Geometry check sheet. Reference: the model listing, model coordinates, mm. Face numbers are marked on the shaded views. A direction names the side the tool comes from. Round coordinates to 2 decimals unless told otherwise and drop trailing zeros. Loops run counter-clockwise (first coordinate to the right, second up) from the corner with the lowest first, then second, coordinate; pieces in that order, holes last. Notation, with made-up numbers: (-13.75, 58.25) - (31.25, 58.25) arc R18 cw to (31.25, 75.25) - close; hole circle Ø11 at (-9, -4.75). An arc over 180 degrees is marked (long way). Answer in a Markdown table with one row per item. Add a question column.
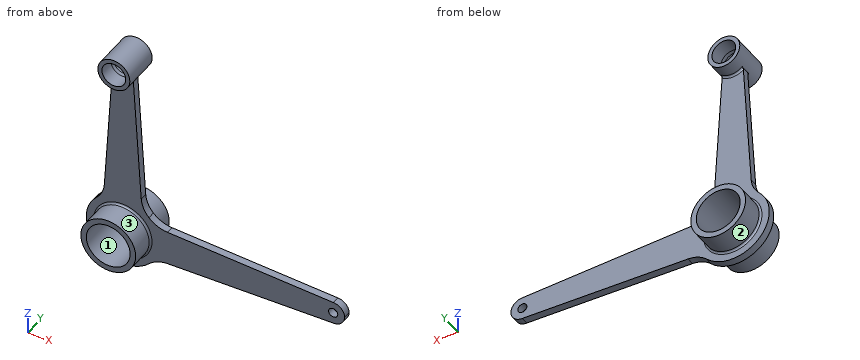
```python
from build123d import *

# Parameters (mm, degrees)
F0_R          = 30
F0_R_2        = 5
F0_R_3        = 13
F1_DEPTH      = 4
F2_R          = 30
F3_T1_DEPTH   = 8
F4_R          = 30
F5_R          = 30
F7_DEPTH      = 20
F6_R          = 30
F6_R_2        = 24
F8_DEPTH      = 30
F9_R          = 2
F10_T4_ANGLE  = 114.9160729666
F10_T10_ANGLE = 114.9160729666


# Not quite as in the source:
# - a fillet or chamfer that OpenCascade refuses, or shapes differently, is made with other operations: its cross-section is extruded or revolved along the edge and cut away or added


with BuildPart() as f1:
    # F0 (on Front) → F1 (new body, symmetric)
    with BuildSketch(Plane.XZ):
        with BuildLine():
            ThreePointArc((34.9249194702, -19.5), (38.7104428986, -10.074800772), (40, 0))
            ThreePointArc((40, 0), (38.7104428986, 10.074800772), (34.9249194702, 19.5))
            ThreePointArc((34.9249194702, 19.5), (28.892590505, 27.6625778609), (21, 34.0440890611))
            ThreePointArc((21, 34.0440890611), (0, 40), (-21, 34.0440890611))
            ThreePointArc((-21, 34.0440890611), (-27.6625778609, -28.892590505), (34.9249194702, -19.5))
        make_face()
        Circle(F0_R, mode=Mode.SUBTRACT)
        with BuildLine():
            ThreePointArc((34.9249194702, 19.5), (38.7104428986, 10.074800772), (40, 0))
            ThreePointArc((40, 0), (38.7104428986, -10.074800772), (34.9249194702, -19.5))
            Line((34.9249194702, -19.5), (230.3062081337, -12.5))
            ThreePointArc((230.3062081337, -12.5), (217.8062081337, 0), (230.3062081337, 12.5))
            Line((230.3062081337, 12.5), (34.9249194702, 19.5))
        make_face()
        with BuildLine():
            ThreePointArc((-21, 34.0440890611), (0, 40), (21, 34.0440890611))
            Line((21, 34.0440890611), (11.5, 186.8090940417))
            ThreePointArc((11.5, 186.8090940417), (0, 182.5), (-11.5, 186.8090940417))
            Line((-11.5, 186.8090940417), (-21, 34.0440890611))
        make_face()
        with BuildLine():
            ThreePointArc((242.8062081337, 0), (239.1450428985, 8.8388347648), (230.3062081337, 12.5))
            ThreePointArc((230.3062081337, 12.5), (217.8062081337, 0), (230.3062081337, -12.5))
            ThreePointArc((230.3062081337, -12.5), (239.1450428985, -8.8388347648), (242.8062081337, 0))
        make_face()
        with Locations((230.3062081337, 0)):
            Circle(F0_R_2, mode=Mode.SUBTRACT)
        with BuildLine():
            ThreePointArc((-11.5, 186.8090940417), (0, 182.5), (11.5, 186.8090940417))
            ThreePointArc((11.5, 186.8090940417), (15.9295323221, 192.7543116269), (17.5, 200))
            ThreePointArc((17.5, 200), (-7.2456883731, 215.9295323221), (-11.5, 186.8090940417))
        make_face()
        with Locations((0, 200)):
            Circle(F0_R_3, mode=Mode.SUBTRACT)
    extrude(amount=F1_DEPTH, both=True)

    # F2
    f2_edges = [f1.edges().sort_by_distance(p)[0] for p in [
        (21, 0, 34.044089),
    ]]
    fillet(f2_edges, radius=F2_R)

    # F3: fillet of radius 30 on 1 edges, made by hand

    # F3_s2 → F3_t1 (join)
    with BuildSketch(Plane.XZ.offset(-4)):
        with BuildLine():
            ThreePointArc((28.5776054959, 27.9878628002), (37.8926630157, 21.5351718891), (48.9366773254, 18.9979954035))
            Line((48.9366773254, 18.9979954035), (34.9249194702, 19.5))
            ThreePointArc((34.9249194702, 19.5), (32.033632685, 23.9550908369), (28.5776054959, 27.9878628002))
        make_face()
    extrude(amount=F3_T1_DEPTH)

    # F4
    f4_edges = [f1.edges().sort_by_distance(p)[0] for p in [
        (-21, 0, 34.044089),
    ]]
    fillet(f4_edges, radius=F4_R)

    # F5
    f5_edges = [f1.edges().sort_by_distance(p)[0] for p in [
        (34.924919, 0, -19.5),
    ]]
    fillet(f5_edges, radius=F5_R)

    # F0 (on Front) → F7 (join, symmetric)
    with BuildSketch(Plane.XZ):
        with BuildLine():
            ThreePointArc((-11.5, 186.8090940417), (0, 182.5), (11.5, 186.8090940417))
            ThreePointArc((11.5, 186.8090940417), (15.9295323221, 192.7543116269), (17.5, 200))
            ThreePointArc((17.5, 200), (-7.2456883731, 215.9295323221), (-11.5, 186.8090940417))
        make_face()
        with Locations((0, 200)):
            Circle(F0_R_3, mode=Mode.SUBTRACT)
    extrude(amount=F7_DEPTH, both=True)

    # F6 (on Front) → F8 (join, symmetric)
    with BuildSketch(Plane.XZ):
        Circle(F6_R)
        Circle(F6_R_2, mode=Mode.SUBTRACT)
    extrude(amount=F8_DEPTH, both=True)

    # F9
    f9_edges = [f1.edges().sort_by_distance(p)[0] for p in [
        (-30, -4, 0),
        (-30, 4, 0),
    ]]
    fillet(f9_edges, radius=F9_R)

    # F10: fillet of radius 2 on 2 edges, made by hand


with BuildPart() as f10_tool2:
    # F10_s3 → F10_t4 (revolve)
    with BuildSketch(Plane(origin=(-90.6925867032, 0, 142.1290246396), x_dir=(0, 1, 0), z_dir=(-0.5379171654, 0, 0.8429977006))):
        with BuildLine():
            ThreePointArc((4, -88.0834330744), (4.5857864376, -89.4976466368), (6, -90.0834330744))
            Line((6, -90.0834330744), (4, -90.0834330744))
            Line((4, -90.0834330744), (4, -88.0834330744))
        make_face()
    revolve(axis=Axis((0, 4, 200), (0, -1, 0)), revolution_arc=F10_T4_ANGLE)

    split(bisect_by=Plane(origin=(-23.028045717, 0, 1.4320454762), x_dir=(0, 1, 0), z_dir=(0.9980719777, 0, -0.0620671193)), keep=Keep.TOP)

    split(bisect_by=Plane(origin=(23.028045717, 0, 1.4320454762), x_dir=(0, 1, 0), z_dir=(-0.9980719777, 0, -0.0620671193)), keep=Keep.TOP)


with BuildPart() as f1_1:
    add(f1.part)

    # F10_t1: union F10_tool2
    add(f10_tool2.part)


with BuildPart() as f10_tool8:
    # F10_s9 → F10_t10 (revolve)
    with BuildSketch(Plane(origin=(90.6925867032, 0, 142.1290246396), x_dir=(0, 1, 0), z_dir=(0.5379171654, 0, 0.8429977006))):
        with BuildLine():
            ThreePointArc((-4, 88.0834330744), (-4.5857864376, 89.4976466368), (-6, 90.0834330744))
            Line((-6, 90.0834330744), (-4, 90.0834330744))
            Line((-4, 90.0834330744), (-4, 88.0834330744))
        make_face()
    revolve(axis=Axis((0, -4, 200), (0, 1, 0)), revolution_arc=F10_T10_ANGLE)

    split(bisect_by=Plane(origin=(-23.028045717, 0, 1.4320454762), x_dir=(0, 1, 0), z_dir=(0.9980719777, 0, -0.0620671193)), keep=Keep.TOP)

    split(bisect_by=Plane(origin=(23.028045717, 0, 1.4320454762), x_dir=(0, 1, 0), z_dir=(-0.9980719777, 0, -0.0620671193)), keep=Keep.TOP)


with BuildPart() as f1_2:
    add(f1_1.part)

    # F10_t7: union F10_tool8
    add(f10_tool8.part)


solid = f1_2.part
```
Q1. Depth check by flat-ended pin: P1, Ø1.5, axis at y = 23, z = 0.5, coming from the +X side; P2, Ø4, axis at x = 197.5, z = 9, coming from the -Y side; P3, Ø12, axis at x = 78, y = 2.5, coming from the -Z side. Enter the tip coordinate at first touch or a pass-through.
Q2. Set-up check for the marked faces 1, 2 and 3: record each of +Z, -Z, +X, -X, +Y, -Y from which the full face is reachable in a straight line by a thin tool's end or side.
Q3. Scan lines: line 1 (Z direction, x = 0, y = -2); line 2 (Z direction, x = 0, y = 14); line 3 (Y direction, x = 4, z = 61.5). Record each from-to range of solid material in increasing order. Write a range as from..to.
Q4. Cross-section at C-C, the plane y = 14. Enter the section's corners in (x, z), plus the area to 3 significant figures.
Q5. Cross-section at B-B, the plane z = 200. Enter the section's corners in (x, y).
Q6. Cross-section at D-D, the plane y = -26. Enter the section's corners in (x, z).
Q7. Cross-section at A-A, the plane x = 0. State how many separate pieces and enclosed holes the cut face has, plus the area to 3 significant figures.
Check sheet entries:
| question | item | result |
|---|---|---|
| 1 | P1 | x = 30 |
| 1 | P2 | y = -4 |
| 1 | P3 | z = -18.17 |
| 2 | face 1 | +Y, -Y |
| 2 | face 2 | +Y |
| 2 | face 3 | -Y |
| 3 | line 1 | -40..-24, 24..187, 213..217.5 |
| 3 | line 2 | -30..-24, 24..30, 182.5..187, 213..217.5 |
| 3 | line 3 | -4..4 |
| 4 | outline | circle Ø60 at (0, 0); circle Ø35 at (0, 200); hole circle Ø48 at (0, 0); hole circle Ø26 at (0, 200) |
| 4 | area | 1,450 mm² |
| 5 | outline | (-17.5, -20) - (-13, -20) - (-13, 20) - (-17.5, 20) - close; (13, -20) - (17.5, -20) - (17.5, 20) - (13, 20) - close |
| 6 | outline | circle Ø60 at (0, 0); hole circle Ø48 at (0, 0) |
| 7 | separate pieces | 3 |
| 7 | enclosed holes | 0 |
| 7 | area | 2,390 mm² |
